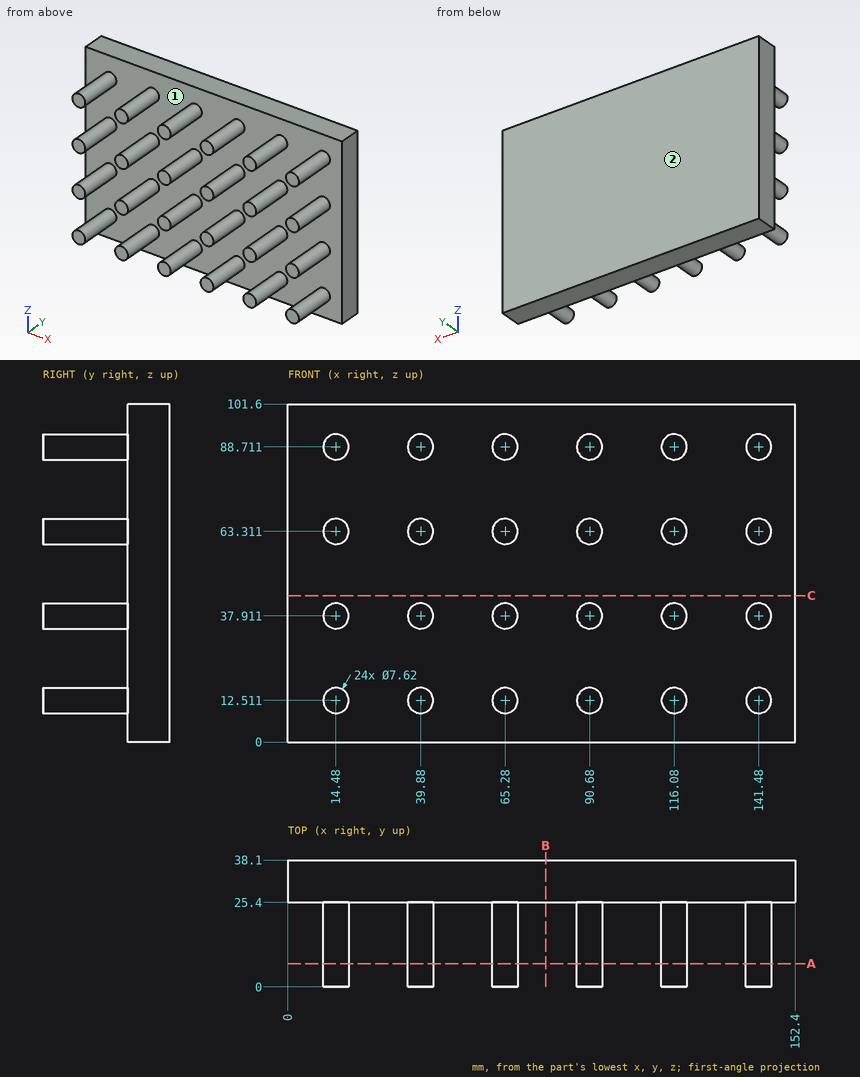
Geometry: see drawing. Coordinates: mm, zero at the bounding-box minimum. Give positions to 0.01 mm unless a question says otherwise; leave off trailing zeros. Order: outer loops, then holes, each group sorted by start corner. A loop starts at its lowest first (then second) coordinate and runs counter-clockwise, first axis right, second up.
Q1. Draft query along Z for the marked faces 1 and 2. Return one class per face: +Z half, -Z half, draft (parallel to the pull), parting line (faces both ways), or undercut.
Checked values:
face 1: undercut
face 2: draft
Q2. Section A-A on y = 7. State how many separate pieces and enclosed holes the cut face has, and give its area (3 significant figures).
Checked values:
separate pieces: 24
enclosed holes: 0
area: 1,090 mm2
Q3. Section C-C on z = 44. Output: boundary loops of the cut face in (x, y).
Checked values:
outline: (0, 25.4) - (152.4, 25.4) - (152.4, 38.1) - (0, 38.1) - close
Q4. Section B-B on x = 77.5. Output: boundary loops of the cut face in (y, z), and give its area (3 significant figures).
Checked values:
outline: (25.4, 0) - (38.1, 0) - (38.1, 101.6) - (25.4, 101.6) - close
area: 1,290 mm2
Q5. Contact query for flat-ended pins moving along their axis: pin 1 Ø2 at (y, z) = (11.5, 34) entering from +X; pin 2 Ø2 at (y, z) = (17.5, 63.5) entering from -X. Output: stop coordinate, or through.
Checked values:
pin 1: stops at x = 143.94
pin 2: stops at x = 10.67
Q6. Ray query, probe 1 along X at (y, z) = (21, 91) (1 decimal); probe 2 along X at (y, z) = (25, 60.5); probe 3 along Y at (x, z) = (106, 89.5). Return the intervals inside material, ascending.
Checked values:
probe 1: x = 11.4 to 17.5, 36.8 to 42.9, 62.2 to 68.3, 87.6 to 93.7, 113 to 119.1, 138.4 to 144.5
probe 2: x = 11.91 to 17.05, 37.31 to 42.45, 62.71 to 67.85, 88.11 to 93.25, 113.51 to 118.65, 138.91 to 144.05
probe 3: y = 25.4 to 38.1
